For this review, take the finished solid that the model builds, in its own axes (mm). A direction names the side the tool comes from. Coordinates: 2 decimals unless noted, no trailing zeros. Loops run counter-clockwise (first coordinate to the right, second up) from the corner with the lowest first, then second, coordinate; pieces in that order, holes last. Notation, with made-up numbers: (-4.75, -32.5) - (17.25, -32.5) arc R16 cw to (17.25, -2.5) - close; hole circle Ø7 at (-39.75, 15.25). An arc over 180 degrees is marked (long way). Answer as a JSON object with one key per item and string values. Group by question number.
Item 1: Tool access review of faces 1 (the cylindrical face through (71.14, 14.63, -149.18)), 2 (the flat face through (50, 53, -95.25)), 3 (the cylindrical face through (98.38, 10.77, -111.74)): name each direction out of +Z, -Z, +X, -X, +Y, -Y from which nothing blocks a thin tool from reaching the whole face with its end or side.
Item 2: We need section D-D (y = 38). Give the boundary of the cut face in (x, z).
Item 3: We need section B-B (y = 19.05). Give the boundary of the cut face in (x, z), then the cut area to 3 significant figures.
Item 4: Clearance check with flat-ended pins moving along their axes: pin 1 (7.5 mm diameter, centred on x = 43.18, y = 88.9, fed in from -Z); pin 2 (5 mm diameter, centred on y = 88.9, z = -124.46, fed in from -X); pin 3 (5.5 mm diameter, centred on x = 43.18, y = 43.18, fed in from -Z). State where each tip first meets the part, or that it passes through.
Item 5: We need section C-C (x = 73.66). State how many separate pieces and enclosed holes the cut face has, then the cut area to 3 significant figures.
Item 6: To check wall thickness, follow line 1 (Z direction, x = 31.5, y = 87.5); line 2 (Y direction, x = 41, z = -112); line 3 (X direction, y = 47.5, z = -74). State the ranges of each line that lie inside material, in increasing order.
Item 7: We need section A-A (z = -31). Give the boundary of the cut face in (x, y).
from build123d import *

# Parameters (mm, degrees)
SKETCH1_W               = 101.6
SKETCH1_H               = 152.4
BOSS_EXTRUDE1_DEPTH     = 101.6
SKETCH3_W               = 88.9
SKETCH3_H               = 139.7
CUT_EXTRUDE1_DEPTH      = 95.25
SKETCH4_W               = 88.9
SKETCH4_H               = 6.35
BOSS_EXTRUDE2_DEPTH     = 95.25
SKETCH6_R               = 3.175
CUT_EXTRUDE2_DEPTH      = 207.448256229
SKETCH7_R               = 3.175
CUT_EXTRUDE3_DEPTH      = 207.448256229
CUT_EXTRUDE5_DEPTH      = 210.453765781
CUT_EXTRUDE5_DEPTH_BACK = 6.35
SKETCH8_R               = 3.175
SKETCH9_W               = 101.6
SKETCH9_H               = 152.4
BOSS_EXTRUDE3_DEPTH     = 6.35
SKETCH10_R              = 6.35
CUT_EXTRUDE6_DEPTH      = 6.35


with BuildPart() as part:
    # Sketch1 → Boss-Extrude1 (new body)
    with BuildSketch(Plane(origin=(0, 0, 0), x_dir=(1, 0, 0), z_dir=(0, 1, 0))):
        with Locations((50.8, 76.2)):
            Rectangle(SKETCH1_W, SKETCH1_H)
    extrude(amount=BOSS_EXTRUDE1_DEPTH)

    # Sketch3 → Cut-Extrude1 (cut)
    with BuildSketch(Plane(origin=(0, 101.6, 0), x_dir=(1, 0, 0), z_dir=(0, 1, 0))):
        with Locations((50.8, 76.2)):
            Rectangle(SKETCH3_W, SKETCH3_H)
    extrude(amount=-CUT_EXTRUDE1_DEPTH, mode=Mode.SUBTRACT)

    # Sketch4 → Boss-Extrude2 (add)
    with BuildSketch(Plane(origin=(0, 6.35, 0), x_dir=(1, 0, 0), z_dir=(0, 1, 0))):
        with Locations((50.8, 98.425)):
            Rectangle(SKETCH4_W, SKETCH4_H)
    extrude(amount=BOSS_EXTRUDE2_DEPTH)

    # Sketch6 → Cut-Extrude2 (cut, through all)
    with BuildSketch(Plane.ZY.offset(-95.25)):
        with Locations((-139.7, 12.7)):
            Circle(SKETCH6_R)
        with Locations((-124.46, 12.7)):
            Circle(SKETCH6_R)
        with Locations((-109.22, 12.7)):
            Circle(SKETCH6_R)
        with Locations((-124.46, 27.94)):
            Circle(SKETCH6_R)
        with Locations((-109.22, 27.94)):
            Circle(SKETCH6_R)
        with Locations((-124.46, 43.18)):
            Circle(SKETCH6_R)
        with Locations((-109.22, 43.18)):
            Circle(SKETCH6_R)
        with Locations((-124.46, 58.42)):
            Circle(SKETCH6_R)
        with Locations((-109.22, 58.42)):
            Circle(SKETCH6_R)
        with Locations((-124.46, 73.66)):
            Circle(SKETCH6_R)
        with Locations((-109.22, 73.66)):
            Circle(SKETCH6_R)
        with Locations((-124.46, 88.9)):
            Circle(SKETCH6_R)
        with Locations((-109.22, 88.9)):
            Circle(SKETCH6_R)
        with Locations((-139.7, 27.94)):
            Circle(SKETCH6_R)
        with Locations((-139.7, 43.18)):
            Circle(SKETCH6_R)
        with Locations((-139.7, 58.42)):
            Circle(SKETCH6_R)
        with Locations((-139.7, 73.66)):
            Circle(SKETCH6_R)
        with Locations((-139.7, 88.9)):
            Circle(SKETCH6_R)
    extrude(amount=-CUT_EXTRUDE2_DEPTH, mode=Mode.SUBTRACT)

    # Sketch7 → Cut-Extrude3 (cut, through all)
    with BuildSketch(Plane(origin=(6.35, 0, 0), x_dir=(0, 0, -1), z_dir=(1, 0, 0))):
        with Locations(Location((139.7, 12.7, 0), (0, 0, 180))):
            Circle(SKETCH7_R)
        with Locations(Location((124.46, 12.7, 0), (0, 0, 180))):
            Circle(SKETCH7_R)
        with Locations(Location((109.22, 12.7, 0), (0, 0, 180))):
            Circle(SKETCH7_R)
        with Locations(Location((124.46, 27.94, 0), (0, 0, 180))):
            Circle(SKETCH7_R)
        with Locations(Location((109.22, 27.94, 0), (0, 0, 180))):
            Circle(SKETCH7_R)
        with Locations(Location((124.46, 43.18, 0), (0, 0, 180))):
            Circle(SKETCH7_R)
        with Locations(Location((109.22, 43.18, 0), (0, 0, 180))):
            Circle(SKETCH7_R)
        with Locations(Location((124.46, 58.42, 0), (0, 0, 180))):
            Circle(SKETCH7_R)
        with Locations(Location((109.22, 58.42, 0), (0, 0, 180))):
            Circle(SKETCH7_R)
        with Locations(Location((124.46, 73.66, 0), (0, 0, 180))):
            Circle(SKETCH7_R)
        with Locations(Location((109.22, 73.66, 0), (0, 0, 180))):
            Circle(SKETCH7_R)
        with Locations(Location((124.46, 88.9, 0), (0, 0, 180))):
            Circle(SKETCH7_R)
        with Locations(Location((109.22, 88.9, 0), (0, 0, 180))):
            Circle(SKETCH7_R)
        with Locations(Location((139.7, 27.94, 0), (0, 0, 180))):
            Circle(SKETCH7_R)
        with Locations(Location((139.7, 43.18, 0), (0, 0, 180))):
            Circle(SKETCH7_R)
        with Locations(Location((139.7, 58.42, 0), (0, 0, 180))):
            Circle(SKETCH7_R)
        with Locations(Location((139.7, 73.66, 0), (0, 0, 180))):
            Circle(SKETCH7_R)
        with Locations(Location((139.7, 88.9, 0), (0, 0, 180))):
            Circle(SKETCH7_R)
    extrude(amount=-CUT_EXTRUDE3_DEPTH, mode=Mode.SUBTRACT)

    # Sketch8 → Cut-Extrude5 (cut, two sides: drawn at the far end of the back side and taken through both)
    with BuildSketch(Plane(origin=(0, 0, -152.4), x_dir=(-1, 0, 0), z_dir=(0, 0, -1)).offset(-CUT_EXTRUDE5_DEPTH_BACK)):
        with Locations(Location((-88.9, 12.7, 0), (0, 0, 180))):
            Circle(SKETCH8_R)
        with Locations(Location((-73.66, 12.7, 0), (0, 0, 180))):
            Circle(SKETCH8_R)
        with Locations(Location((-58.42, 12.7, 0), (0, 0, 180))):
            Circle(SKETCH8_R)
        with Locations(Location((-43.18, 12.7, 0), (0, 0, 180))):
            Circle(SKETCH8_R)
        with Locations(Location((-27.94, 12.7, 0), (0, 0, 180))):
            Circle(SKETCH8_R)
        with Locations(Location((-12.7, 12.7, 0), (0, 0, 180))):
            Circle(SKETCH8_R)
        with Locations(Location((-73.66, 27.94, 0), (0, 0, 180))):
            Circle(SKETCH8_R)
        with Locations(Location((-58.42, 27.94, 0), (0, 0, 180))):
            Circle(SKETCH8_R)
        with Locations(Location((-43.18, 27.94, 0), (0, 0, 180))):
            Circle(SKETCH8_R)
        with Locations(Location((-27.94, 27.94, 0), (0, 0, 180))):
            Circle(SKETCH8_R)
        with Locations(Location((-12.7, 27.94, 0), (0, 0, 180))):
            Circle(SKETCH8_R)
        with Locations(Location((-73.66, 43.18, 0), (0, 0, 180))):
            Circle(SKETCH8_R)
        with Locations(Location((-58.42, 43.18, 0), (0, 0, 180))):
            Circle(SKETCH8_R)
        with Locations(Location((-43.18, 43.18, 0), (0, 0, 180))):
            Circle(SKETCH8_R)
        with Locations(Location((-27.94, 43.18, 0), (0, 0, 180))):
            Circle(SKETCH8_R)
        with Locations(Location((-12.7, 43.18, 0), (0, 0, 180))):
            Circle(SKETCH8_R)
        with Locations(Location((-73.66, 58.42, 0), (0, 0, 180))):
            Circle(SKETCH8_R)
        with Locations(Location((-58.42, 58.42, 0), (0, 0, 180))):
            Circle(SKETCH8_R)
        with Locations(Location((-43.18, 58.42, 0), (0, 0, 180))):
            Circle(SKETCH8_R)
        with Locations(Location((-27.94, 58.42, 0), (0, 0, 180))):
            Circle(SKETCH8_R)
        with Locations(Location((-12.7, 58.42, 0), (0, 0, 180))):
            Circle(SKETCH8_R)
        with Locations(Location((-73.66, 73.66, 0), (0, 0, 180))):
            Circle(SKETCH8_R)
        with Locations(Location((-58.42, 73.66, 0), (0, 0, 180))):
            Circle(SKETCH8_R)
        with Locations(Location((-43.18, 73.66, 0), (0, 0, 180))):
            Circle(SKETCH8_R)
        with Locations(Location((-27.94, 73.66, 0), (0, 0, 180))):
            Circle(SKETCH8_R)
        with Locations(Location((-12.7, 73.66, 0), (0, 0, 180))):
            Circle(SKETCH8_R)
        with Locations(Location((-73.66, 88.9, 0), (0, 0, 180))):
            Circle(SKETCH8_R)
        with Locations(Location((-58.42, 88.9, 0), (0, 0, 180))):
            Circle(SKETCH8_R)
        with Locations(Location((-43.18, 88.9, 0), (0, 0, 180))):
            Circle(SKETCH8_R)
        with Locations(Location((-27.94, 88.9, 0), (0, 0, 180))):
            Circle(SKETCH8_R)
        with Locations(Location((-12.7, 88.9, 0), (0, 0, 180))):
            Circle(SKETCH8_R)
        with Locations(Location((-88.9, 27.94, 0), (0, 0, 180))):
            Circle(SKETCH8_R)
        with Locations(Location((-88.9, 43.18, 0), (0, 0, 180))):
            Circle(SKETCH8_R)
        with Locations(Location((-88.9, 58.42, 0), (0, 0, 180))):
            Circle(SKETCH8_R)
        with Locations(Location((-88.9, 73.66, 0), (0, 0, 180))):
            Circle(SKETCH8_R)
        with Locations(Location((-88.9, 88.9, 0), (0, 0, 180))):
            Circle(SKETCH8_R)
    extrude(amount=CUT_EXTRUDE5_DEPTH + CUT_EXTRUDE5_DEPTH_BACK, mode=Mode.SUBTRACT)

    # Sketch9 → Boss-Extrude3 (add)
    with BuildSketch(Plane(origin=(0, 101.6, 0), x_dir=(1, 0, 0), z_dir=(0, 1, 0))):
        with Locations((50.8, 76.2)):
            Rectangle(SKETCH9_W, SKETCH9_H)
    extrude(amount=BOSS_EXTRUDE3_DEPTH)

    # Sketch10 → Cut-Extrude6 (cut)
    with BuildSketch(Plane(origin=(0, 0, -6.35), x_dir=(-1, 0, 0), z_dir=(0, 0, -1))):
        with Locations((-82.55, 19.05)):
            Circle(SKETCH10_R)
    extrude(amount=-CUT_EXTRUDE6_DEPTH, mode=Mode.SUBTRACT)


solid = part.part
Check sheet entries:
{
 "1": {"face 1": "-Z", "face 2": "none", "face 3": "+X, -X"},
 "2": {"outline": "(0, -152.4) - (101.6, -152.4) - (101.6, 0) - (0, 0) - close; hole (6.35, -146.05) - (95.25, -146.05) - (95.25, -101.6) - (6.35, -101.6) - close; hole (6.35, -95.25) - (95.25, -95.25) - (95.25, -6.35) - (6.35, -6.35) - close"},
 "3": {"outline": "(0, -152.4) - (101.6, -152.4) - (101.6, 0) - (88.9, 0) - (88.9, -6.35) - (95.25, -6.35) - (95.25, -95.25) - (6.35, -95.25) - (6.35, -6.35) - (76.2, -6.35) - (76.2, 0) - (0, 0) - close; hole (6.35, -146.05) - (95.25, -146.05) - (95.25, -101.6) - (6.35, -101.6) - close", "area": "3,550 mm2"},
 "4": {"pin 1": "stops at z = -152.4", "pin 2": "passes through", "pin 3": "stops at z = -101.6"},
 "5": {"separate pieces": "6", "enclosed holes": "1", "area": "3,510 mm2"},
 "6": {"line 1": "z = -152.4 to -146.05, -101.6 to -95.25, -6.35 to 0", "line 2": "y = 0 to 6.35, 101.6 to 107.95", "line 3": "x = 0 to 6.35, 95.25 to 101.6"},
 "7": {"outline": "(0, 0) - (101.6, 0) - (101.6, 107.95) - (0, 107.95) - close; hole (6.35, 6.35) - (95.25, 6.35) - (95.25, 101.6) - (6.35, 101.6) - close"}
}
